```python
from build123d import *

# Parameters (mm, degrees)
BOSS_EXTRUDE1_DEPTH = 10


with BuildPart() as part:
    # Sketch1 → Boss-Extrude1 (new, symmetric)
    with BuildSketch(Plane.XY):
        with BuildLine():
            Line((8, 8.075), (2.9, 8.075))
            Line((2.9, 8.075), (2.9, -1.725))
            ThreePointArc((2.9, -1.725), (2.211700936, -3.386700936), (0.55, -4.075))
            Line((0.55, -4.075), (-0.65, -4.075))
            ThreePointArc((-0.65, -4.075), (-2.311700936, -3.386700936), (-3, -1.725))
            Line((-3, -1.725), (-3, 8.075))
            Line((-3, 8.075), (-8, 8.075))
            Line((-8, 8.075), (-8, 16.075))
            Line((-8, 16.075), (8, 16.075))
            Line((8, 16.075), (8, 8.075))
        make_face()
    extrude(amount=BOSS_EXTRUDE1_DEPTH, both=True)


solid = part.part
```
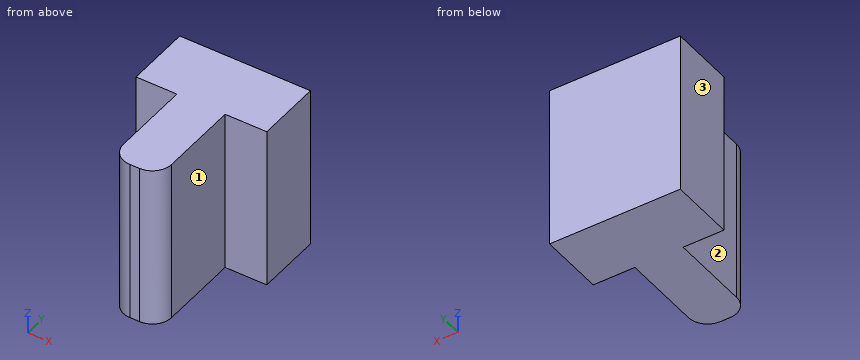
Design review of the part built by this model. Coordinates are the model's own, in mm. Face numbers are marked on the shaded views. A direction names the side the tool comes from. Coordinates: 2 decimals unless noted, no trailing zeros. Order: outer loops, then holes, each group sorted by start corner. A loop starts at its lowest first (then second) coordinate and runs counter-clockwise, first axis right, second up. Notation, with made-up numbers: M -39.5,17 L -35.5,17 A31 ccw -35.5,43 Z; hole C -14.75,9.25 d5. An arc over 180 degrees is marked long. Answer as a JSON object with one key per item and string values. Group by question number.
1) Tool access review of the marked faces 1, 2 and 3: name each direction out of +Z, -Z, +X, -X, +Y, -Y from which nothing blocks a thin tool from reaching the whole face with its end or side.
2) Add section B-B, the plane x = 4.75. Write out the cut boundary in (y, z) (3 decimals), then the cut area to 3 significant figures.
3) For pin 1 (8 mm diameter, centred on y = 2.5, z = 5, fed in from +X); pin 2 (5.5 mm diameter, centred on x = 4.5, z = 3.5, fed in from -Y); pin 3 (1 mm diameter, centred on y = 1.5, z = -1, fed in from -X), all flat-tipped, find the tip position at first contact; note any pin that passes through.
4) Wall thickness on L1, parallel to Y at x = 3.75, z = 8.75 (3 decimals); L2, parallel to X at y = 7, z = 6.75; L3, parallel to Y at x = 1.25, z = -4.5 (3 decimals): over which ranges is each line inside the solid? List them lowest first.
5) Add section C-C, the plane y = -1. Write out the cut boundary in (x, z).
6) Add section A-A, the plane z = 6.25. Write out the cut boundary in (x, y) (3 decimals), then the cut area to 3 significant figures.
Computed values:
{
 "1": {"face 1": "+Z, -Z, +X, -Y", "face 2": "+Z, -Z, -X, -Y", "face 3": "+Z, -Z, -X, +Y, -Y"},
 "2": {"outline": "M 8.075,-10 L 16.075,-10 L 16.075,10 L 8.075,10 Z", "area": "160 mm^2"},
 "3": {"pin 1": "stops at x = 2.9", "pin 2": "stops at y = -3.75", "pin 3": "stops at x = -3"},
 "4": {"L1": "y = 8.075 to 16.075", "L2": "x = -3 to 2.9", "L3": "y = -3.968 to 16.075"},
 "5": {"outline": "M -3,-10 L 2.9,-10 L 2.9,10 L -3,10 Z"},
 "6": {"outline": "M -8,8.075 L -3,8.075 L -3,-1.725 A2.35 ccw -0.65,-4.075 L 0.55,-4.075 A2.35 ccw 2.9,-1.725 L 2.9,8.075 L 8,8.075 L 8,16.075 L -8,16.075 Z", "area": "197 mm^2"}
}
